The listing builds one solid part. Answer for the finished solid, in the listing's coordinates (mm). A direction names the side the tool comes from. Coordinates: 2 decimals unless noted, no trailing zeros. Order: outer loops, then holes, each group sorted by start corner. A loop starts at its lowest first (then second) coordinate and runs counter-clockwise, first axis right, second up. Notation, with made-up numbers: (-26.5, 77.25) -> (9.5, 77.25) arc R29 cw to (9.5, 107.25) -> close; hole circle Ø4 at (33.5, -32.5). An arc over 180 degrees is marked (long way). Answer in a Markdown table with one row per item.
```python
from build123d import *

# Parameters (mm, degrees)
PAD_DEPTH = 7.45
FILLET_R  = 1


with BuildPart() as part:
    # Sketch → Pad (new body)
    with BuildSketch(Plane.XY):
        Polygon((0, 0), (27.2, 0), (27.2, 15.7), (29.7, 15.7), (29.7, 31.7), (27.2, 31.7), (27.2, 18.7), (0, 18.7), (0, 31.7), (-2.5, 31.7), (-2.5, 15.7), (0, 15.7), align=None)
    extrude(amount=PAD_DEPTH)

    # Fillet
    fillet_edges = [part.edges().sort_by_distance(p)[0] for p in [
        (0, 18.7, 3.725),
        (0, 31.7, 3.725),
        (-2.5, 31.7, 3.725),
        (27.2, 31.7, 3.725),
        (29.7, 31.7, 3.725),
        (29.7, 15.7, 3.725),
        (27.2, 18.7, 3.725),
        (-2.5, 15.7, 3.725),
        (0, 15.7, 3.725),
        (27.2, 15.7, 3.725),
    ]]
    fillet(fillet_edges, radius=FILLET_R)


solid = part.part
```
(1) For a pull along X with two mould halves and no side action, classify faces 4 (the flat face through (13, 13, 0)), 5 (the flat face through (27.2, 25, 4)), 6 (the cylindrical face through (-2.199, 31.415, 3.777)) as released by +X, released by -X, zero draft, split by the parting line, or undercut.
Check values:
| item | result |
|---|---|
| face 4 | zero draft |
| face 5 | undercut |
| face 6 | released by -X |
(2) Find the intervals of material crossed by line 1 along X through (y, z) = (28, 5.5); line 2 along Y through (x, z) = (20, 2.25); line 3 along X through (y, z) = (4, 6.5), in increasing order. Write a range as from..to.
Check values:
| item | result |
|---|---|
| line 1 | -2.5..0, 27.2..29.7 |
| line 2 | 0..18.7 |
| line 3 | 0..27.2 |
(3) Flat-ended cylindrical pins translate along their axes: pin 1 (1.5 mm diameter, centred on y = 12, z = 3, fed in from +X); pin 2 (2 mm diameter, centred on x = 16, z = 5, fed in from +Y); pin 3 (3 mm diameter, centred on x = 3, y = 27.5, fed in from -Z). Find the tip coordinate at first contact, or state that the pin passes through.
Check values:
| item | result |
|---|---|
| pin 1 | x = 27.2 |
| pin 2 | y = 18.7 |
| pin 3 | through |
(4) A cutting plane is placed at A-A, the plane y = 21.5. Determine the outline of the cut face in (x, z), then the cut area to 4 significant figures.
Check values:
| item | result |
|---|---|
| outline | (-2.5, 0) -> (0, 0) -> (0, 7.45) -> (-2.5, 7.45) -> close; (27.2, 0) -> (29.7, 0) -> (29.7, 7.45) -> (27.2, 7.45) -> close |
| area | 37.25 mm² |
(5) Which of the six approach directions +Z, -Z, +X, -X, +Y, -Y give full straight-line access (tool end or side, diameter ignored) to faces 1 (the flat face through (27.2, 7, 4)), 2 (the flat face through (29.7, 24, 4)), 3 (the cylindrical face through (26.915, 19.001, 3.777))?
Check values:
| item | result |
|---|---|
| face 1 | +Z, -Z, +X, -Y |
| face 2 | +Z, -Z, +X, +Y, -Y |
| face 3 | +Z, -Z, +Y |
(6) A cutting plane is placed at B-B, the plane z = 2.5. Determine the outline of the cut face in (x, y), then the cut area to 3 significant figures.
Check values:
| item | result |
|---|---|
| outline | (-2.5, 16.7) arc R1 ccw to (-1.5, 15.7) -> (-1, 15.7) arc R1 cw to (0, 14.7) -> (0, 0) -> (27.2, 0) -> (27.2, 14.7) arc R1 cw to (28.2, 15.7) -> (28.7, 15.7) arc R1 ccw to (29.7, 16.7) -> (29.7, 30.7) arc R1 ccw to (28.7, 31.7) -> (28.2, 31.7) arc R1 ccw to (27.2, 30.7) -> (27.2, 19.7) arc R1 cw to (26.2, 18.7) -> (1, 18.7) arc R1 cw to (0, 19.7) -> (0, 30.7) arc R1 ccw to (-1, 31.7) -> (-1.5, 31.7) arc R1 ccw to (-2.5, 30.7) -> close |
| area | 588 mm² |
(7) A cutting plane is placed at C-C, the plane x = 23. Determine the outline of the cut face in (y, z), then the cut area to 3 significant figures.
Check values:
| item | result |
|---|---|
| outline | (0, 0) -> (18.7, 0) -> (18.7, 7.45) -> (0, 7.45) -> close |
| area | 139 mm² |
(8) A cutting plane is placed at D-D, the plane y = 13.5. Determine the outline of the cut face in (x, z).
Check values:
| item | result |
|---|---|
| outline | (0, 0) -> (27.2, 0) -> (27.2, 7.45) -> (0, 7.45) -> close |
